Could you check a few things on this model? Use its own coordinates, in mm. A direction names the side the tool comes from. Give positions to 0.01 mm unless a question says otherwise; leave off trailing zeros. Loops run counter-clockwise (first coordinate to the right, second up) from the corner with the lowest first, then second, coordinate; pieces in that order, holes last. Notation, with made-up numbers: (75.5, 79.25) - (118.5, 79.25) arc R17 ccw to (118.5, 95.25) - close; hole circle Ø5 at (-29.5, 80.5). An arc over 180 degrees is marked (long way). Answer in a Markdown table with one row per item. Add a question column.
```python
from build123d import *

# Parameters (mm, degrees)
SKETCH1_R           = 29
SKETCH1_R_2         = 2.25
SKETCH1_R_3         = 10.25
BOSS_EXTRUDE1_DEPTH = 5
SKETCH4_R           = 11.75
SKETCH4_R_2         = 10.25
BOSS_EXTRUDE2_DEPTH = 1.5
SKETCH12_R          = 3.25
CUT_EXTRUDE5_DEPTH  = 5
SKETCH13_W          = 118.6352657
SKETCH13_H          = 76.236501847
CUT_EXTRUDE6_DEPTH  = 5
CUT_EXTRUDE7_DEPTH  = 5
FILLET2_R           = 3
SKETCH15_R          = 1.5
CUT_EXTRUDE8_DEPTH  = 10
CIRPATTERN1_COUNT   = 6
BOSS_EXTRUDE3_DEPTH = 5
FILLET3_R           = 3


with BuildPart() as part:
    # Sketch1 → Boss-Extrude1 (new body)
    with BuildSketch(Plane(origin=(0, 0, 0), x_dir=(1, 0, 0), z_dir=(0, 1, 0))):
        with BuildLine():
            Line((39.5, 0), (25.25, 100))
            ThreePointArc((25.25, 100), (0, 125.25), (-25.25, 100))
            Line((-25.25, 100), (-39.5, 0))
            ThreePointArc((-39.5, 0), (0, -39.5), (39.5, 0))
        make_face()
        with Locations(Location((0, 0, 0), (0, 0, 270))):
            Circle(SKETCH1_R, mode=Mode.SUBTRACT)
        with Locations(Location((33, 0, 0), (0, 0, 270))):
            Circle(SKETCH1_R_2, mode=Mode.SUBTRACT)
        with Locations(Location((16.5, -28.578838325, 0), (0, 0, 270))):
            Circle(SKETCH1_R_2, mode=Mode.SUBTRACT)
        with Locations(Location((-16.5, -28.578838325, 0), (0, 0, 270))):
            Circle(SKETCH1_R_2, mode=Mode.SUBTRACT)
        with Locations(Location((-33, 0, 0), (0, 0, 270))):
            Circle(SKETCH1_R_2, mode=Mode.SUBTRACT)
        with Locations(Location((0, 100, 0), (0, 0, 270))):
            Circle(SKETCH1_R_3, mode=Mode.SUBTRACT)
    extrude(amount=BOSS_EXTRUDE1_DEPTH)

    # Sketch4 → Boss-Extrude2 (add)
    with BuildSketch(Plane(origin=(0, 5, 0), x_dir=(1, 0, 0), z_dir=(0, 1, 0))):
        with Locations(Location((0, 100, 0), (0, 0, 270))):
            Circle(SKETCH4_R)
        with Locations(Location((0, 100, 0), (0, 0, 270))):
            Circle(SKETCH4_R_2, mode=Mode.SUBTRACT)
    extrude(amount=BOSS_EXTRUDE2_DEPTH)

    # Sketch12 → Cut-Extrude5 (cut)
    with BuildSketch(Plane(origin=(0, 5, 0), x_dir=(1, 0, 0), z_dir=(0, 1, 0))):
        with Locations(Location((28.125255984, 34.496453628, 0), (0, 0, 270))):
            Circle(SKETCH12_R)
        with Locations(Location((26.331961895, 46.867148689, 0), (0, 0, 270))):
            Circle(SKETCH12_R)
        with Locations(Location((24.538667806, 59.237843751, 0), (0, 0, 270))):
            Circle(SKETCH12_R)
        with Locations(Location((22.745373716, 71.608538813, 0), (0, 0, 270))):
            Circle(SKETCH12_R)
    cut_extrude5 = extrude(amount=-CUT_EXTRUDE5_DEPTH, mode=Mode.SUBTRACT)

    # Mirror1: Cut-Extrude5 across plane
    add(cut_extrude5.mirror(Plane(origin=(0, 0, 0), x_dir=(0, 0, 1), z_dir=(1, 0, 0))), mode=Mode.SUBTRACT)

    # Sketch13 → Cut-Extrude6 (cut)
    with BuildSketch(Plane(origin=(0, 5, 0), x_dir=(1, 0, 0), z_dir=(0, 1, 0))):
        with Locations((0, -9.118250923)):
            Rectangle(SKETCH13_W, SKETCH13_H)
    extrude(amount=-CUT_EXTRUDE6_DEPTH, mode=Mode.SUBTRACT)

    # Sketch14 → Cut-Extrude7 (cut)
    with BuildSketch(Plane(origin=(0, 5, 0), x_dir=(1, 0, 0), z_dir=(0, 1, 0))):
        with BuildLine():
            Line((-20.500628763, 29), (20.500628763, 29))
            Line((20.500628763, 29), (12.654649355, 82.31038865))
            ThreePointArc((12.654649355, 82.31038865), (0, 78.25), (-12.654649355, 82.31038865))
            Line((-12.654649355, 82.31038865), (-20.500628763, 29))
        make_face()
    extrude(amount=-CUT_EXTRUDE7_DEPTH, mode=Mode.SUBTRACT)

    # Fillet2
    fillet2_edges = [part.edges().sort_by_distance(p)[0] for p in [
        (-20.500628763, 2.5, -29),
        (-12.654649355, 2.5, -82.31038865),
        (12.654649355, 2.5, -82.31038865),
        (20.500628763, 2.5, -29),
        (35.3675, 2.5, -29),
        (-35.3675, 2.5, -29),
    ]]
    fillet(fillet2_edges, radius=FILLET2_R)

    # Sketch15 → Cut-Extrude8 (cut)
    with BuildSketch(Plane.XZ):
        with Locations(Location((13.5, -100, 0), (0, 0, 270))):
            Circle(SKETCH15_R)
    cut_extrude8 = extrude(amount=-CUT_EXTRUDE8_DEPTH, mode=Mode.SUBTRACT)

    # CirPattern1: Cut-Extrude8 ×6 about axis
    cirpattern1_axis = Axis((0, 0, -100), (0, 1, 0))
    for i in range(1, CIRPATTERN1_COUNT):
        add(cut_extrude8.rotate(cirpattern1_axis, i * 360 / CIRPATTERN1_COUNT), mode=Mode.SUBTRACT)

    # Sketch16 → Boss-Extrude3 (add)
    with BuildSketch(Plane(origin=(0, 5, 0), x_dir=(1, 0, 0), z_dir=(0, 1, 0))):
        with BuildLine():
            ThreePointArc((-19.8904137, 33.146174808), (0, 30.25), (19.8904137, 33.146174808))
            Line((19.8904137, 33.146174808), (18.711950722, 41.153373927))
            ThreePointArc((18.711950722, 41.153373927), (0, 38.25), (-18.711950722, 41.153373927))
            Line((-18.711950722, 41.153373927), (-19.8904137, 33.146174808))
        make_face()
        with BuildLine():
            ThreePointArc((-16.935837694, 53.221373453), (0, 50.25), (16.935837694, 53.221373453))
            Line((16.935837694, 53.221373453), (15.742211816, 61.331598596))
            ThreePointArc((15.742211816, 61.331598596), (0, 58.25), (-15.742211816, 61.331598596))
            Line((-15.742211816, 61.331598596), (-16.935837694, 53.221373453))
        make_face()
    extrude(amount=-BOSS_EXTRUDE3_DEPTH)

    # Fillet3
    fillet3_edges = [part.edges().sort_by_distance(p)[0] for p in [
        (-15.742211816, 2.5, -61.331598596),
        (15.742211816, 2.5, -61.331598596),
        (16.935837694, 2.5, -53.221373453),
        (18.711950722, 2.5, -41.153373927),
        (-18.711950722, 2.5, -41.153373927),
        (19.8904137, 2.5, -33.146174808),
        (-16.935837694, 2.5, -53.221373453),
        (-19.8904137, 2.5, -33.146174808),
    ]]
    fillet(fillet3_edges, radius=FILLET3_R)


solid = part.part
```
(1) We'd pull the mould along Z, two halves only. Please class faces 4 (the flat face through (-28, 3, -29)), 5 (the cylindrical face through (0.19, 2.54, -58.25)), 6 (the cylindrical face through (-14.765, 2.465, -99.194)), 7 (the flat face through (15, 0, -78)): pulls with the +Z half, pulls with the -Z half, needs draft (parallel to the pull), parting line crosses it, or undercut.
(2) For pin 1 Ø1 at (x, y) = (-13, 4) entering from +Z; pin 2 Ø5 at (x, z) = (13.5, -100) entering from +Y; pin 3 Ø10.5 at (x, z) = (24.54, -59.24) entering from +Y, each with a flat end and sliding along its axis, tell me the tip position at first contact or that it passes through.
(3) I want a section at A-A on x = 0. Please give me the cut outline in (y, z).
(4) I want a section at C-C on z = -54. Please give me the cut outline in (x, y) (3 decimals), then the cut area to 3 significant figures.
(5) I want a section at B-B on y = 2. State how many separate pieces and enclosed holes the cut face has, then the cut area to 3 significant figures.
(6) On a 3-axis mill with a long thin cutter (end or side, diameter ignored), from which of +Z, -Z, +X, -X, +Y, -Y can I reach the whole of each face in a straight line? I mean faces 1 (the cylindrical face through (-21.468, 2.465, -29.477)), 2 (the cylindrical face through (-17.89, 2.465, -41.676)), 3 (the flat face through (10, 6.5, -104)). Say none if no direction works.
(7) Please list where these lines run through material, in increasing order: line 1 (X direction, y = 4.5, z = -80); line 2 (Z direction, x = 3, y = 1.5); line 3 (Y direction, x = -5, z = -37).
Reported:
| question | item | result |
|---|---|---|
| 1 | face 4 | pulls with the +Z half |
| 1 | face 5 | undercut |
| 1 | face 6 | undercut |
| 1 | face 7 | needs draft |
| 2 | pin 1 | z = -31.38 |
| 2 | pin 2 | y = 6.5 |
| 2 | pin 3 | y = 5 |
| 3 | outline | (0, -125.25) - (5, -125.25) - (5, -111.75) - (6.5, -111.75) - (6.5, -110.25) - (0, -110.25) - close; (0, -89.75) - (6.5, -89.75) - (6.5, -88.25) - (5, -88.25) - (5, -78.25) - (0, -78.25) - close; (0, -58.25) - (5, -58.25) - (5, -50.25) - (0, -50.25) - close; (0, -38.25) - (5, -38.25) - (5, -30.25) - (0, -30.25) - close |
| 4 | outline | (-31.805, 0) - (31.805, 0) - (31.805, 5) - (-31.805, 5) - close |
| 4 | area | 318 mm² |
| 5 | separate pieces | 1 |
| 5 | enclosed holes | 17 |
| 5 | area | 3,570 mm² |
| 6 | face 1 | +Z, +Y, -Y |
| 6 | face 2 | +Y, -Y |
| 6 | face 3 | +Z, -Z, +X, -X, +Y |
| 7 | line 1 | -28.1 to -12, -8.55 to 8.55, 12 to 28.1 |
| 7 | line 2 | -125.07 to -109.8, -90.2 to -78.46, -58.36 to -50.34, -38.32 to -30.31 |
| 7 | line 3 | 0 to 5 |
